Geometry: final body of the model. Coordinates: model frame, mm. A direction names the side the tool comes from. Give positions to 0.01 mm unless a question says otherwise; leave off trailing zeros. Write each loop counter-clockwise with the first axis right and the second up, starting at its lowest first coordinate (ties: lowest second). Pieces come first, ordered by that corner, then holes. Notation, with made-up numbers: M 69,-7 L 86,-7 A22 ccw 86,26 Z; hole C -14,33 d7. An arc over 180 degrees is marked long. One line per question, with ' | ' between items.
from build123d import *

# Parameters (mm, degrees)
SKETCH1_R           = 40
SKETCH1_R_2         = 26.5
BOSS_EXTRUDE1_DEPTH = 6
SKETCH2_R           = 1.75
CUT_EXTRUDE1_DEPTH  = 7
SKETCH3_R           = 40
SKETCH3_R_2         = 38.5
BOSS_EXTRUDE2_DEPTH = 10


with BuildPart() as part:
    # Sketch1 → Boss-Extrude1 (new body)
    with BuildSketch(Plane.XY):
        Circle(SKETCH1_R)
        Circle(SKETCH1_R_2, mode=Mode.SUBTRACT)
    extrude(amount=BOSS_EXTRUDE1_DEPTH)

    # Sketch2 → Cut-Extrude1 (cut, through all)
    with BuildSketch(Plane.XY.offset(6)):
        with Locations((-31.631941874, 4.839447619)):
            Circle(SKETCH2_R)
        with Locations((4.839447619, 31.631941874)):
            Circle(SKETCH2_R)
        with Locations((31.631941874, -4.839447619)):
            Circle(SKETCH2_R)
        with Locations((-4.839447619, -31.631941874)):
            Circle(SKETCH2_R)
    extrude(amount=-CUT_EXTRUDE1_DEPTH, mode=Mode.SUBTRACT)

    # Sketch3 → Boss-Extrude2 (add)
    with BuildSketch(Plane.XY.offset(6)):
        Circle(SKETCH3_R)
        Circle(SKETCH3_R_2, mode=Mode.SUBTRACT)
    extrude(amount=BOSS_EXTRUDE2_DEPTH)


solid = part.part
(1) Cut plane A-A, the plane y = 0. Return loops of the section in (x, z), then the cut area to 3 significant figures.
Working result:
outline: M -40,0 L -26.5,0 L -26.5,6 L -38.5,6 L -38.5,16 L -40,16 Z; M 26.5,0 L 40,0 L 40,16 L 38.5,16 L 38.5,6 L 26.5,6 Z | area: 192 mm^2
(2) Cut plane C-C, the plane z = 9.25. Return loops of the section in (x, y).
Working result:
outline: C 0,0 d80; hole C 0,0 d77
(3) Draft query along Y for faces 3 (the face through (-9.1, -25.1, 6)), 4 (the face through (26, -8, 0)), 5 (the face through (-8.67, -39.05, 7.89)). Return one class per face: released by +Y, released by -Y, zero draft, split by the parting line, or undercut.
Working result:
face 3: undercut | face 4: zero draft | face 5: split by the parting line
(4) First-contact query: P1, Ø4, axis at y = -20.5, z = 8.5, coming from the +X side; P2, Ø1.5, axis at y = 8, z = 8.5, coming from the +X side; P3, Ø4, axis at y = -12, z = 11.5, coming from the +X side. Flat tips, straight axial feed; report the tip coordinate or a pass-through.
Working result:
P1: stops at x = 35.46 | P2: stops at x = 39.34 | P3: stops at x = 38.73
(5) Set-up query: faces 1 (the face through (14.246, 22.345, 2.958)), 2 (the face through (-30.55, -23.43, 10.93)). Return all of +Z, -Z, +X, -X, +Y, -Y with unobstructed straight access to the full face (end or side cutting, diameter ignored); none if empty.
Working result:
face 1: +Z, -Z | face 2: +Z
(6) Cut plane D-D, the plane z = 3.75. Return loops of the section in (x, y), then the cut area to 3 significant figures.
Working result:
outline: C 0,0 d80; hole C -31.63,4.84 d3.5; hole C 0,0 d53; hole C -4.84,-31.63 d3.5; hole C 4.84,31.63 d3.5; hole C 31.63,-4.84 d3.5 | area: 2,780 mm^2
(7) Material intervals for L1, parallel to Y at x = 0, z = 1.6; L2, parallel to Y at x = -5.5, z = 1.5; L3, parallel to Y at x = -19, z = 3, sorted ascending. Write a range as [from, to].
Working result:
L1: y = [-40, -26.5], [26.5, 40] | L2: y = [-39.62, -33.25], [-30.01, -25.92], [25.92, 39.62] | L3: y = [-35.2, -18.47], [18.47, 35.2]
